Here's how the part is built. I have some questions about the finished solid (model axes, mm). A direction names the side the tool comes from. Round coordinates to 2 decimals unless told otherwise and drop trailing zeros. Loops run counter-clockwise (first coordinate to the right, second up) from the corner with the lowest first, then second, coordinate; pieces in that order, holes last. Notation, with made-up numbers: (-25, 33.5) -> (-6, 33.5) arc R25 cw to (-6, 50.5) -> close; hole circle Ø5 at (-13.75, 29.25). An arc over 180 degrees is marked (long way). Use one line per item in the form item = value. Start each with the question number.
Item 1: For faces 4 (the face through (9.867, 1.989, -75.087)), 5 (the face through (0.246, 23.309, 0.882)), which set-ups out of +Z, -Z, +X, -X, +Y, -Y let a thin tool reach every point of the face, with its end or its side?
Item 2: If we section it at C-C (y = 18): Write out the boundary of the cut face in (x, z), then the cut area to 3 significant figures.
Item 3: If we section it at B-B (x = 17): Write out the boundary of the cut face in (y, z), then the cut area to 3 significant figures.
Item 4: If we section it at A-A (z = -50.5): Write out the boundary of the cut face in (x, y).
Item 5: If I drill on L1, parallel to Y at x = 13.5, z = -62.5; L2, parallel to Z at x = 7.5, y = -3.5; L3, parallel to Z at x = 10.75, y = 1, over which ranges is the centre line in solid material (lowest first)? Write a range as [from, to].
Item 6: Thinking about a two-plate mould opening in Y: for faces 1 (the face through (10, 5, -35)), 2 (the face through (9.87, 1.84, 4.65)), 3 (the face through (0, 6, -19)), which applies, released by +Y, released by -Y, zero draft, split by the parting line, or undercut?
Item 7: I'm going to push flat-ended pins straight in: pin 1 Ø10 at (x, z) = (15, -24) entering from +Y; pin 2 Ø10 at (x, y) = (18, 39) entering from +Z; pin 3 Ø1 at (y, z) = (10, -51.5) entering from +X; pin 4 Ø1 at (x, z) = (15, -15.5) entering from +Y. Where does each tip first touch, or does it pass through?
```python
from build123d import *

# Parameters (mm, degrees)
F1_DEPTH = 20
F2_SIZE  = 0.5


with BuildPart() as f1:
    # F0 (on Right) → F1 (new body)
    with BuildSketch(Plane.YZ):
        with BuildLine():
            ThreePointArc((8, -2.5100299635), (7.3979430927, -3.2935966464), (6.8571428166, -4.1206300966))
            ThreePointArc((6.8571428166, -4.1206300966), (5.4728865379, -7.3422577195), (5, -10.8166538264))
            ThreePointArc((5, -10.8166538264), (5.7729807394, -15.2325342596), (8, -19.1232776893))
            Line((8, -19.1232776893), (8, -10.8166538264))
            Line((8, -10.8166538264), (8, -2.5100299635))
        make_face()
        with BuildLine():
            ThreePointArc((-3.5355339038, 3.5355339081), (1.9134171632, 4.619397662), (5, 0))
            Line((5, 0), (5, -6.2449979984))
            ThreePointArc((5, -6.2449979984), (6.022972164, -5.2653400945), (6.8571428166, -4.1206300966))
            ThreePointArc((6.8571428166, -4.1206300966), (7.7089928828, -2.1380899732), (8, 0))
            ThreePointArc((8, 0), (6.4403338781, 4.7457454145), (2.3694751153, 7.6410462424))
            ThreePointArc((2.3694751153, 7.6410462424), (-1.9198879809, 7.7662107968), (-5.6568542495, 5.6568542495))
            ThreePointArc((-5.6568542495, 5.6568542495), (-4.0221689292, 5.9820133765), (-3.0961940777, 4.5961940777))
            ThreePointArc((-3.0961940777, 4.5961940777), (-3.2103747784, 4.0221689306), (-3.5355339038, 3.5355339081))
        make_face()
        with BuildLine():
            ThreePointArc((-5.6568542495, 5.6568542495), (-5.6568542484, 3.5355339049), (-3.5355339038, 3.5355339081))
            ThreePointArc((-3.5355339038, 3.5355339081), (-3.2103747784, 4.0221689306), (-3.0961940777, 4.5961940777))
            ThreePointArc((-3.0961940777, 4.5961940777), (-4.0221689292, 5.9820133765), (-5.6568542495, 5.6568542495))
        make_face()
        with BuildLine():
            ThreePointArc((8, -70.5), (7.2111025509, -67.0358983849), (5, -64.2550020016))
            Line((5, -64.2550020016), (5, -70.5))
            ThreePointArc((5, -70.5), (1.91341718, -75.119397655), (-3.5355338781, -74.0355339338))
            ThreePointArc((-3.5355338781, -74.0355339338), (-3.2103747714, -74.5221689473), (-3.0961940777, -75.0961940777))
            ThreePointArc((-3.0961940777, -75.0961940777), (-4.0221689259, -76.4820133751), (-5.6568542445, -76.1568542545))
            ThreePointArc((-5.6568542445, -76.1568542545), (3.0614674622, -77.8910362587), (8, -70.5))
        make_face()
        with BuildLine():
            ThreePointArc((-3.5355338781, -74.0355339338), (-5.6568542381, -74.0355338945), (-5.6568542445, -76.1568542545))
            ThreePointArc((-5.6568542445, -76.1568542545), (-4.0221689259, -76.4820133751), (-3.0961940777, -75.0961940777))
            ThreePointArc((-3.0961940777, -75.0961940777), (-3.2103747714, -74.5221689473), (-3.5355338781, -74.0355339338))
        make_face()
        with BuildLine():
            ThreePointArc((6.8571428166, -4.1206300966), (6.022972164, -5.2653400945), (5, -6.2449979984))
            Line((5, -6.2449979984), (5, -10.8166538264))
            ThreePointArc((5, -10.8166538264), (5.4728865379, -7.3422577195), (6.8571428166, -4.1206300966))
        make_face()
        with BuildLine():
            ThreePointArc((21.8503970623, 1.6000463175), (14.3016779708, 1.6461875097), (8, -2.5100299635))
            Line((8, -2.5100299635), (8, -10.8166538264))
            ThreePointArc((8, -10.8166538264), (18, -0.8166538264), (28, -10.8166538264))
            ThreePointArc((28, -10.8166538264), (27.8871906481, -12.3144726031), (27.5513077824, -13.7784977868))
            ThreePointArc((27.5513077824, -13.7784977868), (29.2086767505, -12.7396957014), (30.4840039734, -14.2227743046))
            ThreePointArc((30.4840039734, -14.2227743046), (30.4670825809, -14.4474470536), (30.4167001812, -14.6670507681))
            ThreePointArc((30.4167001812, -14.6670507681), (30.8533478588, -12.7638181291), (31, -10.8166538264))
            ThreePointArc((31, -10.8166538264), (28.4655425519, -3.1048175279), (21.8503970623, 1.6000463175))
        make_face()
        with BuildLine():
            ThreePointArc((27.5513077824, -13.7784977868), (28.5397274827, -15.655470504), (30.4167001812, -14.6670507681))
            ThreePointArc((30.4167001812, -14.6670507681), (30.4670825809, -14.4474470536), (30.4840039734, -14.2227743046))
            ThreePointArc((30.4840039734, -14.2227743046), (29.2086767505, -12.7396957014), (27.5513077824, -13.7784977868))
        make_face()
        with BuildLine():
            ThreePointArc((8, 0), (7.7089928828, -2.1380899732), (6.8571428166, -4.1206300966))
            ThreePointArc((6.8571428166, -4.1206300966), (7.3979430927, -3.2935966464), (8, -2.5100299635))
            Line((8, -2.5100299635), (8, 0))
        make_face()
        with BuildLine():
            ThreePointArc((8, -19.1232776893), (5.7729807394, -15.2325342596), (5, -10.8166538264))
            Line((5, -10.8166538264), (5, -64.2550020016))
            ThreePointArc((5, -64.2550020016), (7.2111025509, -67.0358983849), (8, -70.5))
            Line((8, -70.5), (8, -19.1232776893))
        make_face()
        with BuildLine():
            Line((21.8503970623, 1.6000463175), (2.3694751153, 7.6410462424))
            ThreePointArc((2.3694751153, 7.6410462424), (6.4403338781, 4.7457454145), (8, 0))
            Line((8, 0), (8, -2.5100299635))
            ThreePointArc((8, -2.5100299635), (14.3016779708, 1.6461875097), (21.8503970623, 1.6000463175))
        make_face()
        with BuildLine():
            Line((43.8184051491, -5.2121946824), (21.8503970623, 1.6000463175))
            ThreePointArc((21.8503970623, 1.6000463175), (28.4655425519, -3.1048175279), (31, -10.8166538264))
            ThreePointArc((31, -10.8166538264), (30.8533478588, -12.7638181291), (30.4167001812, -14.6670507681))
            ThreePointArc((30.4167001812, -14.6670507681), (35.3085533829, -8.7807603373), (42.9298518292, -8.0775869762))
            ThreePointArc((42.9298518292, -8.0775869762), (41.9414322781, -6.2006141495), (43.8184051491, -5.2121946824))
        make_face()
        with BuildLine():
            ThreePointArc((44.874128425, -6.6448908094), (44.5816910706, -5.7550636032), (43.8184051491, -5.2121946824))
            ThreePointArc((43.8184051491, -5.2121946824), (41.9414322781, -6.2006141495), (42.9298518292, -8.0775869762))
            ThreePointArc((42.9298518292, -8.0775869762), (44.2639556853, -7.8524534152), (44.874128425, -6.6448908094))
        make_face()
    extrude(amount=F1_DEPTH)

    # F2
    f2_edges = [f1.edges().sort_by_distance(p)[0] for p in [
        (20, -1.919888, 7.766211),
        (20, -5.656854, 3.535534),
        (20, 1.913417, 4.619398),
        (20, 5, -35.25),
        (20, 1.913417, -75.119398),
        (20, -5.656854, -74.035534),
        (20, 3.061467, -77.891036),
        (20, 8, -40.658327),
        (20, 19.497819, -0.929463),
        (20, 28.539727, -15.655471),
        (20, 35.308553, -8.78076),
        (20, 44.806825, -7.089167),
        (20, 23.09394, 1.214426),
        (0, -1.919888, 7.766211),
        (0, -5.656854, 3.535534),
        (0, 1.913417, 4.619398),
        (0, 5, -35.25),
        (0, 1.913417, -75.119398),
        (0, -5.656854, -74.035534),
        (0, 3.061467, -77.891036),
        (0, 8, -40.658327),
        (0, 19.497819, -0.929463),
        (0, 28.539727, -15.655471),
        (0, 35.308553, -8.78076),
        (0, 44.806825, -7.089167),
        (0, 23.09394, 1.214426),
    ]]
    chamfer(f2_edges, length=F2_SIZE)


solid = f1.part
```
Values found:
q1.face_4 = +X, -X
q1.face_5 = +Z, -X, +Y
q2.outline = (0, -0.32) -> (0.5, -0.82) -> (19.5, -0.82) -> (20, -0.32) -> (20, 2.27) -> (19.5, 2.79) -> (0.5, 2.79) -> (0, 2.27) -> close
q2.area = 71.7 mm2
q3.outline = (-5.66, -76.16) arc R8 ccw to (8, -70.5) -> (8, -10.82) arc R10 cw (long way) to (27.55, -13.78) arc R1.5 ccw to (30.42, -14.67) arc R10 cw to (42.93, -8.08) arc R1.5 ccw to (43.82, -5.21) -> (2.37, 7.64) arc R8 ccw to (-5.66, 5.66) arc R1.5 ccw to (-3.54, 3.54) arc R5 cw to (5, 0) -> (5, -70.5) arc R5 cw to (-3.54, -74.04) arc R1.5 ccw to start
q3.area = 550 mm2
q4.outline = (0, 5.5) -> (0.5, 5) -> (19.5, 5) -> (20, 5.5) -> (20, 7.5) -> (19.5, 8) -> (0.5, 8) -> (0, 7.5) -> close
q5.L1 = [5, 8]
q5.L2 = [-77.69, -74.07], [3.57, 7.19]
q5.L3 = [-78.44, -75.4], [4.9, 7.94]
q6.face_1 = released by -Y
q6.face_2 = undercut
q6.face_3 = zero draft
q7.pin_1 = 8
q7.pin_2 = -2.17
q7.pin_3 = through
q7.pin_4 = 30.27
